Source: CAD feature listing. Evaluate the final solid. Frame: model axes, mm. Face numbers are marked on the shaded views. Round coordinates to 2 decimals unless told otherwise and drop trailing zeros. Write each loop counter-clockwise with the first axis right and the second up, starting at its lowest first coordinate (ties: lowest second). Pieces come first, ordered by that corner, then holes.
Autodesk Inventor part; units mm, degrees
ref_plane "YZ Plane" through (0, 0, 0) normal (1, 0, 0) x (0, 1, 0)
ref_plane "XZ Plane" through (0, 0, 0) normal (0, 1, 0) x (-1, 0, 0)
ref_plane "XY Plane" through (0, 0, 0) normal (0, 0, 1) x (1, 0, 0)
sketch "Sketch1" plane through (0, 0, 0) normal (0, 1, 0) x (-1, 0, 0)
  circle A0 centre (0, 0) radius 100
  circle A1 centre (0, 0) radius 90
  circle A2 centre (0, 0) radius 85
  dimension "d0" = 200
  dimension "d1" = 180
  dimension "d2" = 170
extrude "Extrusion1" add sketch "Sketch1" along normal blind 8 contours A0 | A1 | A2
extrude "Extrusion2" add sketch "Sketch1" along normal blind 10
extrude "Extrusion3" add sketch "Sketch1" against normal blind 80 contours A0 | A1 | A2
sketch "Sketch2" plane through (0, 10, 0) normal (0, 1, 0) x (1, 0, 0)
  circle A0 centre (0, -0.8314) radius 75
  point P0 (0, 0)
  dimension "d9" = 150
extrude "Extrusion4" cut sketch "Sketch2" against normal blind 25
sketch "Sketch3" plane through (0, 0, 0) normal (1, 0, 0) x (0, 1, 0)
  line L0 (5.4504, 100.114) -> (0.3612, 91.2991)
  line L1 (5.4504, 100.114) -> (15.629, 100.114) construction
  line L2 (-80, 100) -> (10, 100)
  line L3 (-25, 100) -> (-20.6699, 92.5)
  line L4 (-25, 100) -> (-16.3397, 100) construction
  line L5 (-20.6699, 92.5) -> (1.0545, 92.5)
  line L6 (5.4504, 100.114) -> (-20.6699, 100)
  line L7 (-33.1258, 0) -> (23.7548, 0)
  line L8 (1.0545, 92.5) -> (-70.8596, 92.5)
  line L9 (-70.8596, 92.5) -> (-80, 100)
  point P0 (0, 0)
  point P1 (5.3846, 100)
  dimension "d12" = 120
  dimension "d13" = 60
revolve "Revolution1" cut sketch "Sketch3" angle 360 about axis through (0, -10, 0) along (0, 1, 0) contours L0 L5 L3 L2
sketch "Sketch6" plane through (0, -15, 0.8314) normal (0, 1, 0) x (1, 0, 0)
  circle A0 centre (0, 0.8314) radius 42
  circle A1 centre (-25.5623, 34.1567) radius 1
  circle A2 centre (-16.0794, -37.9688) radius 1
  circle A3 centre (41.6416, 6.3064) radius 1
  circle A4 centre (0, 0.8314) radius 1
  dimension "d32" = 84
  dimension "d33" = 2
  dimension "d36" = 360
  dimension "d40" = 2
extrude "Extrusion7" add sketch "Sketch6" along normal blind 50 contours A3 A0 | A0 A3 | A2 A0 | A0 A2 | A1 A0 | A0 A1 | A4
properties part number "Base"
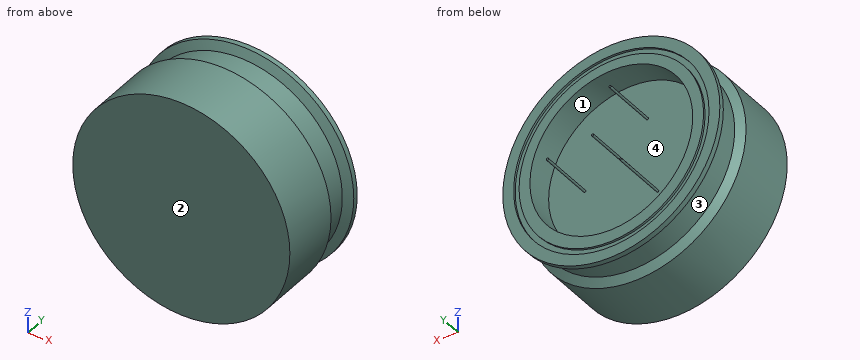
1) Material intervals for line 1 (Z direction, x = 0, y = 9.2); line 2 (X direction, y = 9.25, z = 0); line 3 (X direction, y = -10.5, z = 2), sorted ascending.
Taken from the geometry:
line 1: z = -100 to -90, -85 to -74.17, -1 to 1, 75.83 to 85, 90 to 100
line 2: x = -100 to -90, -85 to -75, -1 to 1, 75 to 85, 90 to 100
line 3: x = -92.48 to -74.99, 74.99 to 92.48
2) Contact query for flat-ended pins moving along their axis: P1, Ø6, axis at y = -40, z = -31, coming from the -X side; P2, Ø4, axis at x = -17, y = -56, coming from the +Z side; P3, Ø4, axis at y = -27.5, z = 50.5, coming from the +X side. Output: stop coordinate, or through.
Taken from the geometry:
P1: stops at x = -96
P2: stops at z = 98.87
P3: stops at x = 87.45
3) Section query C-C on y = 18. Return the cut outline in (x, z) (3 decimals).
Taken from the geometry:
outline: circle Ø2 at (-25.562, -33.325); circle Ø2 at (-16.079, 38.8); circle Ø2 at (0, 0); circle Ø2 at (41.642, -5.475)
4) Section query A-A on y = -10.5. Return the cut outline in (x, z) (3 decimals), then the cut area to 3 significant figures.
Taken from the geometry:
outline: circle Ø185 at (0, 0); circle Ø2 at (-25.562, -33.325); circle Ø2 at (-16.079, 38.8); circle Ø2 at (0, 0); circle Ø2 at (41.642, -5.475); hole circle Ø150 at (0, 0.831)
area: 9,220 mm2
5) Pull-direction query (Y, two-part tool) for the marked faces 1, 2, 3 and 4; classes: released by +Y, released by -Y, zero draft, split by the parting line, or undercut.
Taken from the geometry:
face 1: zero draft
face 2: released by -Y
face 3: undercut
face 4: released by +Y
6) Section query B-B on y = -69. Return the cut outline in (x, z), then the cut area to 3 significant figures.
Taken from the geometry:
outline: circle Ø200 at (0, 0)
area: 31,400 mm2
